Design review of the part built by this model. Coordinates are the model's own, in mm. A direction names the side the tool comes from. Give positions to 0.01 mm unless a question says otherwise; leave off trailing zeros. Order: outer loops, then holes, each group sorted by start corner. A loop starts at its lowest first (then second) coordinate and runs counter-clockwise, first axis right, second up. Notation, with made-up numbers: M -9.5,-0.75 L 1.5,-0.75 A25 ccw 1.5,21.25 Z; hole C 69,86 d7. An arc over 180 degrees is marked long. Answer as a JSON object with one key per item and string values.
from build123d import *

# Parameters (mm, degrees)
F2_T     = -2
F3_R     = 7.5
F3_R_2   = 5.5
F4_DEPTH = 2


with BuildPart() as f1:
    # F0 (on Top) → F1 (revolve)
    with BuildSketch(Plane.XY):
        with BuildLine():
            Line((0, 0), (-7.5, 0))
            ThreePointArc((-7.5, 0), (-5.303301, -5.303301), (0, -7.5))
            Line((0, -7.5), (0, 0))
        make_face()
    revolve(axis=Axis((0, -3.75, 0), (0, -1, 0)))

    # F2
    f2_openings = [f1.faces().sort_by_distance(p)[0] for p in [
        (0, 0, 0),
    ]]
    offset(amount=F2_T, openings=f2_openings)

    # F3 (on face) → F4 (join)
    with BuildSketch(Plane(origin=(0, 0, 0), x_dir=(-1, 0, 0), z_dir=(0, 1, 0))):
        with BuildLine():
            Line((-6.25, -8.75), (6.25, -8.75))
            ThreePointArc((6.25, -8.75), (8.017767, -8.017767), (8.75, -6.25))
            Line((8.75, -6.25), (8.75, 6.25))
            ThreePointArc((8.75, 6.25), (8.017767, 8.017767), (6.25, 8.75))
            Line((6.25, 8.75), (-6.25, 8.75))
            ThreePointArc((-6.25, 8.75), (-8.017767, 8.017767), (-8.75, 6.25))
            Line((-8.75, 6.25), (-8.75, -6.25))
            ThreePointArc((-8.75, -6.25), (-8.017767, -8.017767), (-6.25, -8.75))
        make_face()
        Circle(F3_R, mode=Mode.SUBTRACT)
        Circle(F3_R)
        Circle(F3_R_2, mode=Mode.SUBTRACT)
    extrude(amount=F4_DEPTH)


solid = f1.part
(1) Tool access review of faces 1 (the flat face through (-8, 0, 0)), 2 (the flat face through (0, 1, 8.75)), 3 (the cylindrical face through (1.19, 0.99, -5.37)): name each direction out of +Z, -Z, +X, -X, +Y, -Y from which nothing blocks a thin tool from reaching the whole face with its end or side.
Checked values:
{"face 1": "-Y", "face 2": "+Z, +X, -X, +Y, -Y", "face 3": "+Y"}
(2) To check wall thickness, follow L1, parallel to X at y = 1.1, z = 0; L2, parallel to Y at x = 7.75, z = -0.25. State the ranges of each line that lie inside material, in increasing order. Write a range as from..to.
Checked values:
{"L1": "x = -8.75..-5.5, 5.5..8.75", "L2": "y = 0..2"}
(3) We need section A-A (y = 1). Write out the cut boundary in (x, z).
Checked values:
{"outline": "M -8.75,-6.25 A2.5 ccw -6.25,-8.75 L 6.25,-8.75 A2.5 ccw 8.75,-6.25 L 8.75,6.25 A2.5 ccw 6.25,8.75 L -6.25,8.75 A2.5 ccw -8.75,6.25 Z; hole C 0,0 d11"}
(4) Insertion check: pin 1 (6 mm diameter, centred on x = -5.5, z = 4, fed in from -Y); pin 2 (2 mm diameter, centred on y = 0.5, z = 7, fed in from +X); pin 3 (8 mm diameter, centred on x = -2.5, z = 6, fed in from -Y); pin 4 (5 mm diameter, centred on x = 4.5, z = 1.5, fed in from -Y). Each pin has a flat end and moves straight along its axis. Give the tip position at first contact, or say it passes through.
Checked values:
{"pin 1": "stops at y = -6.47", "pin 2": "stops at x = 8.75", "pin 3": "stops at y = -7.07", "pin 4": "stops at y = -7.16"}
